```python
from build123d import *

# Parameters (mm, degrees)
FILLET2_R               = 5
FILLET3_R               = 5
CUT_EXTRUDE1_DEPTH      = 20
CUT_EXTRUDE1_DEPTH_BACK = 20
SKETCH5_R               = 7.5


with BuildPart() as part:
    # Sketch4 → Revolve1 (revolve)
    with BuildSketch(Plane(origin=(0, 0, 0), x_dir=(0, 0, -1), z_dir=(1, 0, 0)), mode=Mode.PRIVATE) as revolve1_sk:
        Polygon((-215.028448312, -8.762321339), (0, -8.762321339), (0, 8.237678661), (-200.028448312, 8.237678661), (-200.028448312, 21.237678661), (-215.028448312, 21.237678661), align=None)
    revolve(revolve1_sk.sketch.rotate(Axis((0, -8.762321339, 221.52106333), (0, 0, -1)), 90), axis=Axis((0, -8.762321339, 221.52106333), (0, 0, -1)))

    # Fillet2
    fillet2_edges = [part.edges().sort_by_distance(p)[0] for p in [
        (-17, -8.762321339, 0),
    ]]
    fillet(fillet2_edges, radius=FILLET2_R)

    # Fillet3
    fillet3_edges = [part.edges().sort_by_distance(p)[0] for p in [
        (-30, -8.762321339, 215.028448312),
    ]]
    fillet(fillet3_edges, radius=FILLET3_R)

    # Sketch5 → Cut-Extrude1 (cut, two sides: drawn at the far end of the back side and taken through both)
    with BuildSketch(Plane(origin=(0, 0, 0), x_dir=(0, 0, -1), z_dir=(1, 0, 0)).offset(-CUT_EXTRUDE1_DEPTH_BACK)):
        with Locations(Location((-19.67963909, -8.762321339, 0), (0, 0, 180))):
            Circle(SKETCH5_R)
    extrude(amount=CUT_EXTRUDE1_DEPTH + CUT_EXTRUDE1_DEPTH_BACK, mode=Mode.SUBTRACT)


solid = part.part
```
Geometry check sheet. Reference: the model listing, model coordinates, mm. A direction names the side the tool comes from. Coordinates: 2 decimals unless noted, no trailing zeros. Loops run counter-clockwise (first coordinate to the right, second up) from the corner with the lowest first, then second, coordinate; pieces in that order, holes last.
Item 1: Sectioned sample at B-B, the plane z = 17.5. Record the boundary of the cut face in (x, y).
Item 2: Go/stop test with flat-tipped pins: pin 1 Ø1.5 at (x, y) = (-18, -31) entering from +Z; pin 2 Ø12 at (x, z) = (-20, 34) entering from +Y; pin 3 Ø5 at (y, z) = (2, 80.5) entering from -X. Record where each tip stops, or that it passes through.
Item 3: Thickness scan on line 1 (Z direction, x = 8.5, y = -15); line 2 (Y direction, x = -11, z = 26); line 3 (Z direction, x = 22, y = -8). Record the ranges inside material, lowest first.
Item 4: Access from +Z, -Z, +X, -X, +Y, -Y to the whole of each face (thin tool, end or side, straight path). Record for faces 1 (the face through (-13, 4, 200.028)), 2 (the face through (-0.24, -11.02, 26.83)).
Item 5: Sectioned sample at C-C, the plane z = 72. Record the boundary of the cut face in (x, y), then the cut area to 3 significant figures.
Item 6: Sectioned sample at A-A, the plane x = 0. Record the boundary of the cut face in (y, z), then the cut area to 3 significant figures.
Check result:
1. outline: (-15.41, -15.94) arc R17 ccw to (15.41, -15.94) - close; (-15.41, -1.59) - (15.41, -1.59) arc R17 ccw to start
2. pin 1: stops at z = 214.13
2. pin 2: stops at y = 0.88
2. pin 3: stops at x = -14.86
3. line 1: z = 0 to 15.52, 23.84 to 215.03
3. line 2: y = -21.72 to -12.8, -4.72 to 4.2
3. line 3: z = 200.03 to 215.03
4. face 1: -Z
4. face 2: +X, -X
5. outline: circle Ø34 at (0, -8.76)
5. area: 908 mm2
6. outline: (-38.76, 200.03) - (-25.76, 200.03) - (-25.76, 5) arc R5 ccw to (-20.76, 0) - (3.24, 0) arc R5 ccw to (8.24, 5) - (8.24, 200.03) - (21.24, 200.03) - (21.24, 210.03) arc R5 ccw to (16.24, 215.03) - (-33.76, 215.03) arc R5 ccw to (-38.76, 210.03) - close; hole circle Ø15 at (-8.76, 19.68)
6. area: 7,500 mm2
